Read the model definition and answer for the solid it produces. Units are mm, in the model's axes. Face numbers are marked on the shaded views. A direction names the side the tool comes from. Give positions to 0.01 mm unless a question says otherwise; leave off trailing zeros. Order: outer loops, then holes, each group sorted by start corner. A loop starts at its lowest first (then second) coordinate and runs counter-clockwise, first axis right, second up.
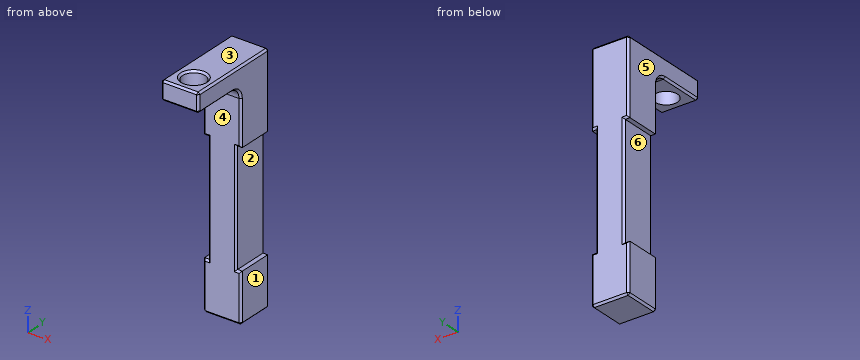
```python
from build123d import *

# Parameters (mm, degrees)
SKETCH1_W            = 10
SKETCH1_H            = 58
BOSS_EXTRUDE1_DEPTH  = 10
CUT_EXTRUDE1_REACH   = 33.081
SKETCH2_W            = 1.25
SKETCH2_H            = 30
SKETCH3_W            = 10
SKETCH3_H            = 25
BOSS_EXTRUDE2_DEPTH  = 5
FILLET1_R            = 3
M5_CLEARANCE_HOLE1_D = 6
CHAMFER1_SIZE        = 0.5


with BuildPart() as part:
    # Sketch1 → Boss-Extrude1 (new body)
    with BuildSketch(Plane(origin=(0, 0, 0), x_dir=(1, 0, 0), z_dir=(0, 1, 0))):
        Rectangle(SKETCH1_W, SKETCH1_H)
    extrude(amount=-BOSS_EXTRUDE1_DEPTH)

    # Sketch2 → Cut-Extrude1 (cut, up to next)
    with BuildSketch(Plane(origin=(0, 0, 0), x_dir=(1, 0, 0), z_dir=(0, 1, 0)), mode=Mode.PRIVATE) as cut_extrude1_sk1:
        with Locations((-4.375, 1)):
            Rectangle(SKETCH2_W, SKETCH2_H)
    cut_extrude1_tool1 = extrude(cut_extrude1_sk1.sketch, amount=-CUT_EXTRUDE1_REACH, mode=Mode.PRIVATE) & part.part
    # Sketch2 → Cut-Extrude1 (cut, up to next)
    with BuildSketch(Plane(origin=(0, 0, 0), x_dir=(1, 0, 0), z_dir=(0, 1, 0)), mode=Mode.PRIVATE) as cut_extrude1_sk2:
        with Locations((4.375, 1)):
            Rectangle(SKETCH2_W, SKETCH2_H)
    cut_extrude1_tool2 = extrude(cut_extrude1_sk2.sketch, amount=-CUT_EXTRUDE1_REACH, mode=Mode.PRIVATE) & part.part
    add(cut_extrude1_tool1.solids().sort_by_distance((-4.375, 0, -1))[0], mode=Mode.SUBTRACT)
    add(cut_extrude1_tool2.solids().sort_by_distance((4.375, 0, -1))[0], mode=Mode.SUBTRACT)

    # Sketch3 → Boss-Extrude2 (add)
    with BuildSketch(Plane.XY.offset(29)):
        with Locations((0, -12.5)):
            Rectangle(SKETCH3_W, SKETCH3_H)
    extrude(amount=BOSS_EXTRUDE2_DEPTH)

    # Fillet1
    fillet1_edges = [part.edges().sort_by_distance(p)[0] for p in [
        (0, -10, 29),
    ]]
    fillet(fillet1_edges, radius=FILLET1_R)

    # M5 Clearance Hole1 (through all)
    with Locations(Plane.XY.offset(34)):
        with Locations((0, -20)):
            Hole(M5_CLEARANCE_HOLE1_D / 2)

    # Chamfer1
    chamfer1_edges = [part.edges().sort_by_distance(p)[0] for p in [
        (-5, -10, -22.5),
        (5, 0, -22.5),
        (-5, 0, 24),
        (5, -10, -22.5),
        (-5, -10, 20),
        (-4.375, -10, -16),
        (-3.75, -10, -1),
        (-4.375, -10, 14),
        (-4.375, 0, 14),
        (-3.75, 0, -1),
        (-4.375, 0, -16),
        (4.375, -10, 14),
        (3.75, -10, -1),
        (4.375, -10, -16),
        (4.375, 0, -16),
        (3.75, 0, -1),
        (4.375, 0, 14),
        (0, -25, 29),
        (-5, -25, 31.5),
        (5, -19, 29),
        (5, -25, 31.5),
        (-5, -12.5, 34),
        (0, -25, 34),
        (5, -12.5, 34),
        (0, 0, 34),
        (-5, 0, -22.5),
        (0, 0, -29),
        (-5, -19, 29),
        (5, -10, 20),
        (5, -10.878679656, 28.121320344),
        (-5, -10.878679656, 28.121320344),
        (5, 0, 24),
        (3, -20, 34),
        (-5, -5, -29),
        (5, -5, -29),
        (0, -10, -29),
    ]]
    chamfer(chamfer1_edges, length=CHAMFER1_SIZE)


solid = part.part
```
1) Consider L1, parallel to Z at x = -4, y = -7.5; L2, parallel to Y at x = 0, z = 30.1; L3, parallel to Y at x = 4.5, z = -21. Determine where each line is inside the solid, lowest interval first.
Final values:
L1: z = -29 to -16, 14 to 34
L2: y = -25 to -23, -17 to 0
L3: y = -10 to 0
2) For a pull along Z with two mould halves and no side action, classify the marked faces 1, 2 and 3 as released by +Z, released by -Z, zero draft, split by the parting line, or undercut.
Final values:
face 1: zero draft
face 2: undercut
face 3: released by +Z
3) A tool of negligible diameter and unlimited length cuts with its end or side. For the marked faces 4, 5 and 6, from which of +Z, -Z, +X, -X, +Y, -Y can it reach the whole face along a straight path? Write none if from no direction.
Final values:
face 4: -Z, +X, -X, -Y
face 5: +Z, -Z, -X, +Y, -Y
face 6: -X, +Y, -Y
4) The part is cut by section D-D on y = -15.5. Determine the outline of the cut face in (x, z).
Final values:
outline: (-5, 29.5) - (-4.5, 29) - (4.5, 29) - (5, 29.5) - (5, 33.5) - (4.5, 34) - (-4.5, 34) - (-5, 33.5) - close
5) The part is cut by section B-B on x = 0. Determine the outline of the cut face in (y, z), and give its area (3 significant figures).
Final values:
outline: (-25, 29.5) - (-24.5, 29) - (-23, 29) - (-23, 33.5) - (-23.5, 34) - (-24.5, 34) - (-25, 33.5) - close; (-17, 29) - (-13, 29) arc R3 cw to (-10, 26) - (-10, -28.5) - (-9.5, -29) - (-0.5, -29) - (0, -28.5) - (0, 33.5) - (-0.5, 34) - (-16.5, 34) - (-17, 33.5) - close
area: 676 mm2
6) The part is cut by section A-A on y = -20. Determine the outline of the cut face in (x, z), and give its area (4 significant figures).
Final values:
outline: (-5, 29.5) - (-4.5, 29) - (-3, 29) - (-3, 33.5) - (-3.5, 34) - (-4.5, 34) - (-5, 33.5) - close; (3, 29) - (4.5, 29) - (5, 29.5) - (5, 33.5) - (4.5, 34) - (3.5, 34) - (3, 33.5) - close
area: 19.25 mm2
7) The part is cut by section C-C on z = -21.5. Determine the outline of the cut face in (x, y), and give its area (3 significant figures).
Final values:
outline: (-5, -9.5) - (-4.5, -10) - (4.5, -10) - (5, -9.5) - (5, -0.5) - (4.5, 0) - (-4.5, 0) - (-5, -0.5) - close
area: 99.5 mm2
8) Given pin 1 (4 mm diameter, centred on x = -1, z = 15, fed in from -Y); pin 2 (10 mm diameter, centred on y = -6.5, z = 5, fed in from -X); pin 3 (1.5 mm diameter, centred on x = -1, y = -17.5, fed in from -Z), each flat-ended and moving along its own axis, determine where each tip first touches the part or whether it passes through.
Final values:
pin 1: stops at y = -10
pin 2: stops at x = -3.75
pin 3: stops at z = 29
